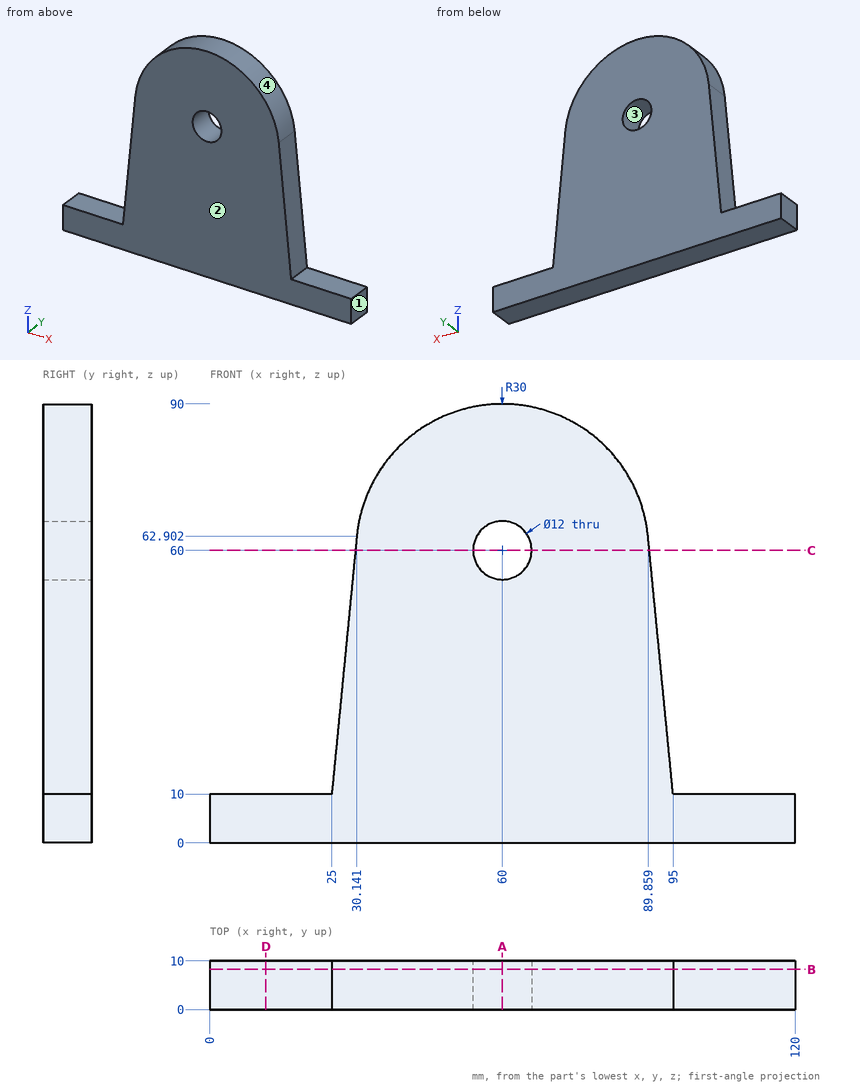
Geometry check sheet. Reference: drawing and pictorial views, mm from the part's lowest x, y, z. Round coordinates to 2 decimals unless told otherwise and drop trailing zeros. Write each loop counter-clockwise with the first axis right and the second up, starting at its lowest first coordinate (ties: lowest second). Pieces come first, ordered by that corner, then holes.
(1) Depth check by flat-ended pin: pin 1 Ø4 at (y, z) = (3.5, 41) entering from -X; pin 2 Ø9.5 at (x, z) = (60, 60) entering from +Y; pin 3 Ø3 at (y, z) = (5, 76) entering from -X; pin 4 Ø4 at (y, z) = (8.5, 63.5) entering from +X (1 decimal). Enter the tip coordinate at first touch or a pass-through.
Returned:
pin 1: stops at x = 27.82
pin 2: passes through
pin 3: stops at x = 33.74
pin 4: stops at x = 90
(2) Section check C-C (z = 60). Enter the section's corners in (x, y), plus the area to 3 significant figures.
Returned:
outline: (29.86, 0) - (54, 0) - (54, 10) - (29.86, 10) - close; (66, 0) - (90.14, 0) - (90.14, 10) - (66, 10) - close
area: 483 mm2
(3) Mould release check, pull along X, two halves, no side actions. Record for the marked faces 1, 2, 3 and 4: pulls with the +X half, pulls with the -X half, needs draft (parallel to the pull), parting line crosses it, or undercut.
Returned:
face 1: pulls with the +X half
face 2: needs draft
face 3: undercut
face 4: parting line crosses it
(4) Section check B-B (y = 8.25). Enter the section's corners in (x, z), plus the area to 3 significant figures.
Returned:
outline: (0, 0) - (120, 0) - (120, 10) - (95, 10) - (89.86, 62.9) arc R30 ccw to (30.14, 62.9) - (25, 10) - (0, 10) - close; hole circle Ø12 at (60, 60)
area: 5,760 mm2
(5) Material ranges on line 1 (Z direction, x = 60, y = 5.75); line 2 (Z direction, x = 6.5, y = 4.5); line 3 (X direction, y = 9.75, z = 61) (1 decimal), recorded low to high.
Returned:
line 1: z = 0 to 54, 66 to 90
line 2: z = 0 to 10
line 3: x = 30 to 54.1, 65.9 to 90
(6) Section check D-D (x = 11.5). Enter the section's corners in (y, z).
Returned:
outline: (0, 0) - (10, 0) - (10, 10) - (0, 10) - close
(7) Section check A-A (x = 60). Enter the section's corners in (y, z).
Returned:
outline: (0, 0) - (10, 0) - (10, 54) - (0, 54) - close; (0, 66) - (10, 66) - (10, 90) - (0, 90) - close
